Build history of the part. All positions in model axes, mm. A direction names the side the tool comes from. Round coordinates to 2 decimals unless told otherwise and drop trailing zeros.
Item 1: Drop a flat-ended pin along its axis: pin 1 Ø5 at (x, z) = (-7.78, -7.78) entering from -Y. Give the stop position or say it passes through.
Item 2: 3-axis set-ups, long thin cutter, end or side, ignore diameter. For faces 1 (the flat face through (0, 1.2, -13)), 2 (the cylindrical face through (12.214, 1.61, -5.853)): which of +Z, -Z, +X, -X, +Y, -Y reach the whole face in a straight line?
Item 3: Wall check: probe 1 along X at (y, z) = (0.45, 0); probe 2 along X at (y, z) = (2.5, 0); probe 3 along Z at (x, y) = (0, 1.5). Give the ranges that are in metal, low to high.
Item 4: Mould opens along Z. For faces 3 (the flat face through (5.2, 0, 5.2)), 4 (the cylindrical face through (-0.35, 2.17, 9.44)) say: +Z half, -Z half, draft (parallel to the pull), parting line (faces both ways), or undercut.
```python
from build123d import *

# Parameters (mm, degrees)
SKETCH1_R           = 25
SKETCH1_R_2         = 7.15
BOSS_EXTRUDE1_DEPTH = 3.175
SKETCH2_R           = 2.25
CUT_EXTRUDE1_DEPTH  = 4.175
CIRPATTERN1_COUNT   = 6
SKETCH4_R           = 1.6
CUT_EXTRUDE3_DEPTH  = 4.175
SKETCH5_R           = 2.7
CUT_EXTRUDE4_DEPTH  = 1.2
CIRPATTERN3_COUNT   = 8
FILLET1_R           = 0.8


with BuildPart() as part:
    # Sketch1 → Boss-Extrude1 (new body)
    with BuildSketch(Plane(origin=(0, 0, 0), x_dir=(1, 0, 0), z_dir=(0, 1, 0))):
        Circle(SKETCH1_R)
        Circle(SKETCH1_R_2, mode=Mode.SUBTRACT)
    extrude(amount=BOSS_EXTRUDE1_DEPTH)

    # Sketch2 → Cut-Extrude1 (cut, through all)
    with BuildSketch(Plane(origin=(0, 3.175, 0), x_dir=(1, 0, 0), z_dir=(0, 1, 0))):
        with Locations((0, 15.5)):
            Circle(SKETCH2_R)
    cut_extrude1 = extrude(amount=-CUT_EXTRUDE1_DEPTH, mode=Mode.SUBTRACT)

    # CirPattern1: Cut-Extrude1 ×6 about axis
    cirpattern1_axis = Axis((0, 0, 0), (0, 1, 0))
    for i in range(1, CIRPATTERN1_COUNT):
        add(cut_extrude1.rotate(cirpattern1_axis, i * 360 / CIRPATTERN1_COUNT), mode=Mode.SUBTRACT)

    # Sketch4 → Cut-Extrude3 (cut, through all)
    with BuildSketch(Plane.XZ):
        with Locations((0, 11)):
            Circle(SKETCH4_R)
    cut_extrude3 = extrude(amount=-CUT_EXTRUDE3_DEPTH, mode=Mode.SUBTRACT)

    # Sketch5 → Cut-Extrude4 (cut)
    with BuildSketch(Plane.XZ):
        with Locations((0, 11)):
            Circle(SKETCH5_R)
    cut_extrude4 = extrude(amount=-CUT_EXTRUDE4_DEPTH, mode=Mode.SUBTRACT)

    # CirPattern3: Cut-Extrude3, Cut-Extrude4 ×8 about axis
    cirpattern3_axis = Axis((0, 0, 0), (0, 1, 0))
    for i in range(1, CIRPATTERN3_COUNT):
        add(cut_extrude3.rotate(cirpattern3_axis, i * 360 / CIRPATTERN3_COUNT), mode=Mode.SUBTRACT)
        add(cut_extrude4.rotate(cirpattern3_axis, i * 360 / CIRPATTERN3_COUNT), mode=Mode.SUBTRACT)

    # Fillet1
    fillet1_edges = [part.edges().sort_by_distance(p)[0] for p in [
        (-25, 3.175, 0),
    ]]
    fillet(fillet1_edges, radius=FILLET1_R)


solid = part.part
```
Results:
1. pin 1: stops at y = 1.2
2. face 1: -Y
2. face 2: +Y, -Y
3. probe 1: x = -25 to -13.7, -8.3 to -7.15, 7.15 to 8.3, 13.7 to 25
3. probe 2: x = -24.99 to -12.6, -9.4 to -7.15, 7.15 to 9.4, 12.6 to 24.99
3. probe 3: z = -25 to -17.75, -13.25 to -12.6, -9.4 to -7.15, 7.15 to 9.4, 12.6 to 13.25, 17.75 to 25
4. face 3: draft
4. face 4: undercut
